Can you work these out from the model? Positions are in its coordinate system, mm. A direction names the side the tool comes from. Give positions to 0.01 mm unless a question says otherwise; leave off trailing zeros. Loops run counter-clockwise (first coordinate to the right, second up) from the corner with the lowest first, then second, coordinate; pieces in that order, holes last. Notation, with made-up numbers: (80, -18.75) - (97, -18.75) arc R33 cw to (97, 18.25) - close; hole circle Ø6 at (42, 42.25). An arc over 180 degrees is marked (long way). Answer as a JSON object with one key per item and string values.
```python
from build123d import *

# Parameters (mm, degrees)
BOSS_EXTRUDE1_DEPTH = 215.9
BOSS_EXTRUDE2_DEPTH = 60


with BuildPart() as part:
    # Sketch1 → Boss-Extrude1 (new, symmetric)
    with BuildSketch(Plane(origin=(0, 0, 0), x_dir=(0, 0, -1), z_dir=(1, 0, 0))):
        Polygon((0, 0), (-21.28355545, 0), (183.928530546, 563.815572472), (202.722382962, 556.975169605), align=None)
    extrude(amount=BOSS_EXTRUDE1_DEPTH, both=True)

    # Sketch2 → Boss-Extrude2 (add)
    with BuildSketch(Plane(origin=(215.9, 0, 0), x_dir=(0, 0, -1), z_dir=(1, 0, 0))):
        with BuildLine():
            Line((-1.717345436, 314.558459548), (9.648049621, 309.258688795))
            Line((9.648049621, 309.258688795), (6.222130729, 325.218973302))
            ThreePointArc((6.222130729, 325.218973302), (0.284125678, 329.058256569), (-3.55515759, 323.120251518))
            Line((-3.55515759, 323.120251518), (-1.717345436, 314.558459548))
        make_face()
        with BuildLine():
            Line((9.648049621, 309.258688795), (79.43330187, 276.717291245))
            Line((79.43330187, 276.717291245), (86.299833965, 295.582933124))
            Line((86.299833965, 295.582933124), (-85.071109517, 375.494516454))
            ThreePointArc((-85.071109517, 375.494516454), (-98.360370005, 370.657621201), (-93.523474752, 357.368360714))
            Line((-93.523474752, 357.368360714), (-1.717345436, 314.558459548))
            Line((-1.717345436, 314.558459548), (-3.55515759, 323.120251518))
            ThreePointArc((-3.55515759, 323.120251518), (0.284125678, 329.058256569), (6.222130729, 325.218973302))
            Line((6.222130729, 325.218973302), (9.648049621, 309.258688795))
        make_face()
        Polygon((39.930228547, 168.18348929), (9.648049621, 309.258688795), (-1.717345436, 314.558459548), (33.496662431, 150.507411661), align=None)
        with BuildLine():
            Line((45.549887934, 142.00325401), (39.930228547, 168.18348929))
            Line((39.930228547, 168.18348929), (33.496662431, 150.507411661))
            Line((33.496662431, 150.507411661), (35.772599615, 139.904532226))
            ThreePointArc((35.772599615, 139.904532226), (41.710604666, 136.065248958), (45.549887934, 142.00325401))
        make_face()
        with BuildLine():
            Line((79.43330187, 276.717291245), (87.738082656, 272.844708365))
            ThreePointArc((87.738082656, 272.844708365), (101.027343143, 277.681603618), (96.19044789, 290.970864106))
            Line((96.19044789, 290.970864106), (86.299833965, 295.582933124))
            Line((86.299833965, 295.582933124), (79.43330187, 276.717291245))
        make_face()
    boss_extrude2 = extrude(amount=BOSS_EXTRUDE2_DEPTH)

    # Mirror1: Boss-Extrude2 across plane
    add(boss_extrude2.mirror(Plane(origin=(0, 0, 0), x_dir=(0, 0, 1), z_dir=(1, 0, 0))))


solid = part.part
```
1) I'm going to push flat-ended pins straight in: P1, Ø12, axis at y = 394.5, z = -146, coming from the -X side; P2, Ø1.5, axis at x = 72, y = 315, coming from the -Z side; P3, Ø6, axis at x = 55.5, y = 501, coming from the -Z side. Where does each tip first touch, or does it pass through?
Check sheet entries:
{"P1": "x = -215.9", "P2": "z = -114.92", "P3": "z = -183.44"}
2) Imagine slicing it at C-C on x = -107. Write out the boundary of the cut face in (y, z).
Check sheet entries:
{"outline": "(0, 0) - (556.98, -202.72) - (563.82, -183.93) - (0, 21.28) - close"}
3) Imagine slicing it at B-B on z = -54.5. Write out the boundary of the cut face in (x, y), and give its area (3 significant figures).
Check sheet entries:
{"outline": "(-275.9, 288.34) - (-215.9, 288.34) - (-215.9, 310.41) - (-275.9, 310.41) - close; (-215.9, 149.74) - (215.9, 149.74) - (215.9, 208.21) - (-215.9, 208.21) - close; (215.9, 288.34) - (275.9, 288.34) - (275.9, 310.41) - (215.9, 310.41) - close", "area": "27,900 mm2"}
4) Imagine slicing it at A-A on y = 327. Write out the boundary of the cut face in (x, z), and give its area (3 significant figures).
Check sheet entries:
{"outline": "(-275.9, -18.93) - (-215.9, -18.93) - (-215.9, 28.4) - (-275.9, 28.4) - close; (-215.9, -119.02) - (215.9, -119.02) - (215.9, -97.73) - (-215.9, -97.73) - close; (215.9, -18.93) - (275.9, -18.93) - (275.9, 28.4) - (215.9, 28.4) - close", "area": "14,900 mm2"}
5) Which directions (+Z, -Z, +X, -X, +Y, -Y) give clear straight access to the entire face, cutting with the end or side of a thin tool? Please do faces 1 (the flat face through (-215.9, 306, -7)), 2 (the flat face through (3, 0, 10)).
Check sheet entries:
{"face 1": "+Z, +Y", "face 2": "+Z, -Z, +X, -X, -Y"}
6) I need wall thicknesses on L1, parallel to X at y = 221, z = -64; L2, parallel to Z at x = -111, y = 109; L3, parallel to Z at x = -132, y = 295.5. Which ranges of each line are inside material? Lowest first, please.
Check sheet entries:
{"L1": "-215.9 to 215.9", "L2": "-39.67 to -18.39", "L3": "-107.55 to -86.27"}
7) Imagine slicing it at D-D on z = -112.5. Write out the boundary of the cut face in (x, y), and give its area (4 significant figures).
Check sheet entries:
{"outline": "(-215.9, 309.09) - (215.9, 309.09) - (215.9, 367.57) - (-215.9, 367.57) - close", "area": "25,250 mm2"}
